```python
from build123d import *

# Parameters (mm, degrees)
ESQUISSE1_W             = 12.7
ESQUISSE1_H             = 42.5
ESQUISSE1_R             = 1.6
BOSS_EXTRU_1_DEPTH      = 4
ESQUISSE2_W             = 4.9
ESQUISSE2_H             = 42.5
BOSS_EXTRU_2_DEPTH      = 15
ENL_V_MAT_EXTRU_1_DEPTH = 5.9
CHANFREIN1_SIZE         = 10


with BuildPart() as part:
    # Esquisse1 → Boss.-Extru.1 (new body)
    with BuildSketch(Plane.XY):
        with Locations((32.265489842, 21.249999998)):
            Rectangle(ESQUISSE1_W, ESQUISSE1_H)
        with Locations((34.615489842, 3.999999998)):
            Circle(ESQUISSE1_R, mode=Mode.SUBTRACT)
        with Locations((34.615489842, 38.499999998)):
            Circle(ESQUISSE1_R, mode=Mode.SUBTRACT)
    extrude(amount=BOSS_EXTRU_1_DEPTH)

    # Esquisse2 → Boss.-Extru.2 (add)
    with BuildSketch(Plane.XY.offset(4)):
        with Locations((28.365489842, 21.249999998)):
            Rectangle(ESQUISSE2_W, ESQUISSE2_H)
    extrude(amount=BOSS_EXTRU_2_DEPTH)

    # Esquisse3 → Enlèv. mat.-Extru.1 (cut, through all)
    with BuildSketch(Plane(origin=(30.815489842, 0, 0), x_dir=(0, 0, -1), z_dir=(1, 0, 0))):
        with BuildLine():
            Line((-13, 27.250000431), (-19, 27.250000431))
            Line((-19, 27.250000431), (-19, 15.250000431))
            Line((-19, 15.250000431), (-13, 15.250000431))
            ThreePointArc((-13, 15.250000431), (-7, 21.250000431), (-13, 27.250000431))
        make_face()
    extrude(amount=-ENL_V_MAT_EXTRU_1_DEPTH, mode=Mode.SUBTRACT)

    # Chanfrein1
    chanfrein1_edges = [part.edges().sort_by_distance(p)[0] for p in [
        (28.365489842, 42.499999998, 19),
        (28.365489842, -2e-09, 19),
    ]]
    chamfer(chanfrein1_edges, length=CHANFREIN1_SIZE)


solid = part.part
```
Geometry: final body of the model. Coordinates: model frame, mm. A direction names the side the tool comes from. Round coordinates to 2 decimals unless told otherwise and drop trailing zeros. Order: outer loops, then holes, each group sorted by start corner. A loop starts at its lowest first (then second) coordinate and runs counter-clockwise, first axis right, second up. Notation, with made-up numbers: M -20.75,40.5 L 13.25,40.5 A34 ccw 13.25,75.5 Z; hole C -38.75,63.25 d8. An arc over 180 degrees is marked long. Use one line per item in the form item = value. Start each with the question number.
Q1. Cut plane B-B (z = 17). Return loops of the section in (x, y), and give its area (4 significant figures).
Q2. Access query for faces 1 (the face through (35, 22, 4)), 2 (the face through (33.017, 38.57, 1.972)). Directions: +Z, -Z, +X, -X, +Y, -Y. A direction counts if a zero-diameter tool reaches every point of the face in a straight line with its end or side. Return the directions, or none.
Q3. Cut plane C-C (x = 33.75). Return loops of the section in (y, z).
Q4. Cut plane A-A (y = 38.5). Return loops of the section in (x, z).
Q5. Pin query (flat end, axial travel): pin 1 Ø1.5 at (x, z) = (28.5, 15.5) entering from +Y; pin 2 Ø2.5 at (x, z) = (28.5, 15) entering from -Y; pin 3 Ø3.5 at (x, y) = (34.62, 4) entering from +Z; pin 4 Ø1.9 at (x, y) = (34.62, 38.5) entering from +Z. Return the tip coordinate at first contact, or that it passes through.
Q6. Mould query, pull axis Y, two halves, no side actions, for faces 3 (the face through (30.815, 21, 6)), 4 (the face through (28, 27.25, 16)), 5 (the face through (28, 15.25, 16)), 6 (the face through (28.3, 37.4, 14.1)). Classes: +Y half, -Y half, draft (parallel to the pull), parting line (faces both ways), or undercut.
Q7. Material intervals for line 1 (X direction, y = 38.5, z = 1.65); line 2 (X direction, y = 38, z = 5.5); line 3 (Z direction, x = 33.25, y = 5), sorted ascending. Write a range as [from, to].
Q8. Cut plane D-D (x = 27.25). Return loops of the section in (y, z), and give its area (3 significant figures).
Geometry results:
q1.outline = M 25.92,8 L 30.82,8 L 30.82,15.25 L 25.92,15.25 Z; M 25.92,27.25 L 30.82,27.25 L 30.82,34.5 L 25.92,34.5 Z
q1.area = 71.05 mm^2
q2.face_1 = +Z, +X, +Y, -Y
q2.face_2 = +Z, -Z
q3.outline = M 0,0 L 2.65,0 L 2.65,4 L 0,4 Z; M 5.35,0 L 37.15,0 L 37.15,4 L 5.35,4 Z; M 39.85,0 L 42.5,0 L 42.5,4 L 39.85,4 Z
q4.outline = M 25.92,0 L 33.02,0 L 33.02,4 L 30.82,4 L 30.82,13 L 25.92,13 Z; M 36.22,0 L 38.62,0 L 38.62,4 L 36.22,4 Z
q5.pin_1 = 36.75
q5.pin_2 = 4.75
q5.pin_3 = 4
q5.pin_4 = through
q6.face_3 = draft
q6.face_4 = undercut
q6.face_5 = undercut
q6.face_6 = +Y half
q7.line_1 = [25.92, 33.02], [36.22, 38.62]
q7.line_2 = [25.92, 30.82]
q7.line_3 = [0, 4]
q8.outline = M 0,0 L 42.5,0 L 42.5,9 L 32.5,19 L 27.25,19 L 27.25,13 A6 cw 15.25,13 L 15.25,19 L 10,19 L 0,9 Z
q8.area = 579 mm^2
